Verification items for the finished model (mm, model axes). Face numbers are marked on the shaded views. A direction names the side the tool comes from. Give positions to 0.01 mm unless a question says otherwise; leave off trailing zeros. Loops run counter-clockwise (first coordinate to the right, second up) from the corner with the lowest first, then second, coordinate; pieces in that order, holes last. Notation, with made-up numbers: (59, 17) -> (75, 17) arc R24 cw to (75, 49) -> close; hole circle Ø2 at (-19, 4.5). An arc over 180 degrees is marked (long way). Answer in a Markdown table with one row per item. Add a question column.
Q1. Section check D-D on z = -42.5. Enter the section's corners in (x, y), and give its area (3 significant figures).
Q2. Section check A-A on y = -44. Enter the section's corners in (x, z), and give its area (3 significant figures).
Q3. Gauge pin test, flat ends, axial feed: P1, Ø12.5, axis at x = 45, y = 13, coming from the -Z side; P2, Ø18, axis at y = -16, z = 41, coming from the +X side; P3, Ø3.5, axis at x = 0, y = -15, coming from the -Z side; P4, Ø12, axis at y = 11.5, z = -4, coming from the -X side. Record the tip position at first contact, or that the pin passes through.
Q4. Section check B-B on z = 1. Enter the section's corners in (x, y), and give its area (3 significant figures).
Q5. Material ranges on probe 1 along Y at (x, z) = (0, -79); probe 2 along Y at (x, z) = (0, -78.85); probe 3 along Z at (x, y) = (-43, 4), recorded low to high.
Q6. Release check for a two-part mould opening along X. For the marked faces 5 and 6 record: pulls with the +X half, pulls with the -X half, needs draft (parallel to the pull), parting line crosses it, or undercut.
Q7. Section check C-C on x = -75. Enter the section's corners in (y, z), and give its area (3 significant figures).
Q8. Set-up check for the marked faces 1, 2, 3 and 4: record each of +Z, -Z, +X, -X, +Y, -Y from which the full face is reachable in a straight line by a thin tool's end or side.
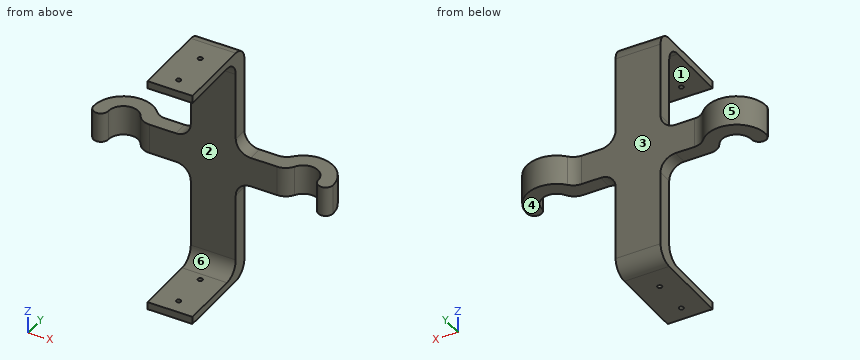
```python
from build123d import *

# Parameters (mm, degrees)
BOSS_EXTRUDE1_DEPTH     = 10
SKETCH2_W               = 30
SKETCH2_H               = 160.5
BOSS_EXTRUDE2_DEPTH     = 10
SKETCH3_W               = 30
SKETCH3_H               = 5
BOSS_EXTRUDE3_DEPTH     = 50
SKETCH4_R               = 1.5
CUT_EXTRUDE1_DEPTH      = 1
CUT_EXTRUDE1_DEPTH_BACK = 161.5
FILLET1_R               = 10
FILLET2_R               = 10
FILLET3_R               = 10


with BuildPart() as part:
    # Sketch1 → Boss-Extrude1 (new body, symmetric)
    with BuildSketch(Plane.XY):
        with BuildLine():
            ThreePointArc((-70, 0), (-60, 10), (-50, 0))
            Line((-50, 0), (-40, 0))
            ThreePointArc((-40, 0), (-40.681483474, 5.176380902), (-42.679491924, 10))
            ThreePointArc((-42.679491924, 10), (-65.176380902, 19.318516526), (-80, 0))
            ThreePointArc((-80, 0), (-75, -5), (-70, 0))
        make_face()
        with BuildLine():
            ThreePointArc((-42.679491924, 10), (-40.681483474, 5.176380902), (-40, 0))
            Line((-40, 0), (40, 0))
            ThreePointArc((40, 0), (40.681483474, 5.176380902), (42.679491924, 10))
            Line((42.679491924, 10), (-42.679491924, 10))
        make_face()
        with BuildLine():
            ThreePointArc((42.679491924, 10), (40.681483474, 5.176380902), (40, 0))
            Line((40, 0), (50, 0))
            ThreePointArc((50, 0), (60, 10), (70, 0))
            ThreePointArc((70, 0), (75, -5), (80, 0))
            ThreePointArc((80, 0), (65.176380902, 19.318516526), (42.679491924, 10))
        make_face()
    extrude(amount=BOSS_EXTRUDE1_DEPTH, both=True)

    # Sketch2 → Boss-Extrude2 (add)
    with BuildSketch(Plane.XZ):
        Rectangle(SKETCH2_W, SKETCH2_H)
    extrude(amount=-BOSS_EXTRUDE2_DEPTH)

    # Sketch3 → Boss-Extrude3 (add)
    with BuildSketch(Plane.XZ):
        with Locations((0, 77.75)):
            Rectangle(SKETCH3_W, SKETCH3_H)
    boss_extrude3 = extrude(amount=BOSS_EXTRUDE3_DEPTH)

    # Mirror1: Boss-Extrude3 across plane
    add(boss_extrude3.mirror(Plane.XY))

    # Sketch4 → Cut-Extrude1 (cut, two sides)
    with BuildSketch(Plane.XY.offset(80.25)) as cut_extrude1_sk:
        with Locations((0, -40)):
            Circle(SKETCH4_R)
        with Locations((0, -15)):
            Circle(SKETCH4_R)
    extrude(amount=CUT_EXTRUDE1_DEPTH, mode=Mode.SUBTRACT)
    extrude(cut_extrude1_sk.sketch, amount=-CUT_EXTRUDE1_DEPTH_BACK, mode=Mode.SUBTRACT)

    # Fillet1
    fillet1_edges = [part.edges().sort_by_distance(p)[0] for p in [
        (0, 10, -80.25),
        (0, 10, 80.25),
        (0, 0, 75.25),
        (0, 0, -75.25),
    ]]
    fillet(fillet1_edges, radius=FILLET1_R)

    # Fillet2
    fillet2_edges = [part.edges().sort_by_distance(p)[0] for p in [
        (-15, 5, -10),
        (15, 5, -10),
        (15, 5, 10),
        (-15, 5, 10),
    ]]
    fillet(fillet2_edges, radius=FILLET2_R)

    # Fillet3
    fillet3_edges = [part.edges().sort_by_distance(p)[0] for p in [
        (-42.679491924, 10, 0),
        (42.679491924, 10, 0),
        (50, 0, 0),
        (-50, 0, 0),
    ]]
    fillet(fillet3_edges, radius=FILLET3_R)


solid = part.part
```
Taken from the geometry:
| question | item | result |
|---|---|---|
| 1 | outline | (-15, 0) -> (15, 0) -> (15, 10) -> (-15, 10) -> close |
| 1 | area | 300 mm² |
| 2 | outline | (-15, -80.25) -> (15, -80.25) -> (15, -75.25) -> (-15, -75.25) -> close; (-15, 75.25) -> (15, 75.25) -> (15, 80.25) -> (-15, 80.25) -> close |
| 2 | area | 300 mm² |
| 3 | P1 | stops at z = -10 |
| 3 | P2 | passes through |
| 3 | P3 | stops at z = -80.25 |
| 3 | P4 | stops at x = -79.23 |
| 4 | outline | (-80, 0) arc R5 ccw to (-70, 0) arc R10 cw to (-51.34, 5) arc R10 ccw to (-42.68, 0) -> (42.68, 0) arc R10 ccw to (51.34, 5) arc R10 cw to (70, 0) arc R5 ccw to (80, 0) arc R20 ccw to (45.09, 13.33) arc R10 cw to (37.64, 10) -> (-37.64, 10) arc R10 cw to (-45.09, 13.33) arc R20 ccw to start |
| 4 | area | 1,830 mm² |
| 5 | probe 1 | y = -50 to -41.5, -38.5 to -16.5, -13.5 to 4.84 |
| 5 | probe 2 | y = -50 to -41.5, -38.5 to -16.5, -13.5 to 5.1 |
| 5 | probe 3 | z = -10 to 10 |
| 6 | face 5 | undercut |
| 6 | face 6 | needs draft |
| 7 | outline | (-5, -10) -> (13.23, -10) -> (13.23, 10) -> (-5, 10) -> close |
| 7 | area | 365 mm² |
| 8 | face 1 | +X, -X, -Y |
| 8 | face 2 | -Y |
| 8 | face 3 | +Z, -Z, +Y |
| 8 | face 4 | -Z, +X, +Y, -Y |
